Check sheet for the drawn part. Datum: minimum x, y, z corner. Units: mm. Round coordinates to 2 decimals unless told otherwise and drop trailing zeros. Order: outer loops, then holes, each group sorted by start corner. A loop starts at its lowest first (then second) coordinate and runs counter-clockwise, first axis right, second up. Notation, with made-up numbers: (-16, 65) -> (-8, 65) arc R25 ccw to (-8, 82) -> close; hole circle Ø11 at (62.5, 76.5). An arc over 180 degrees is marked (long way). Answer in a Markdown table with one row per item.
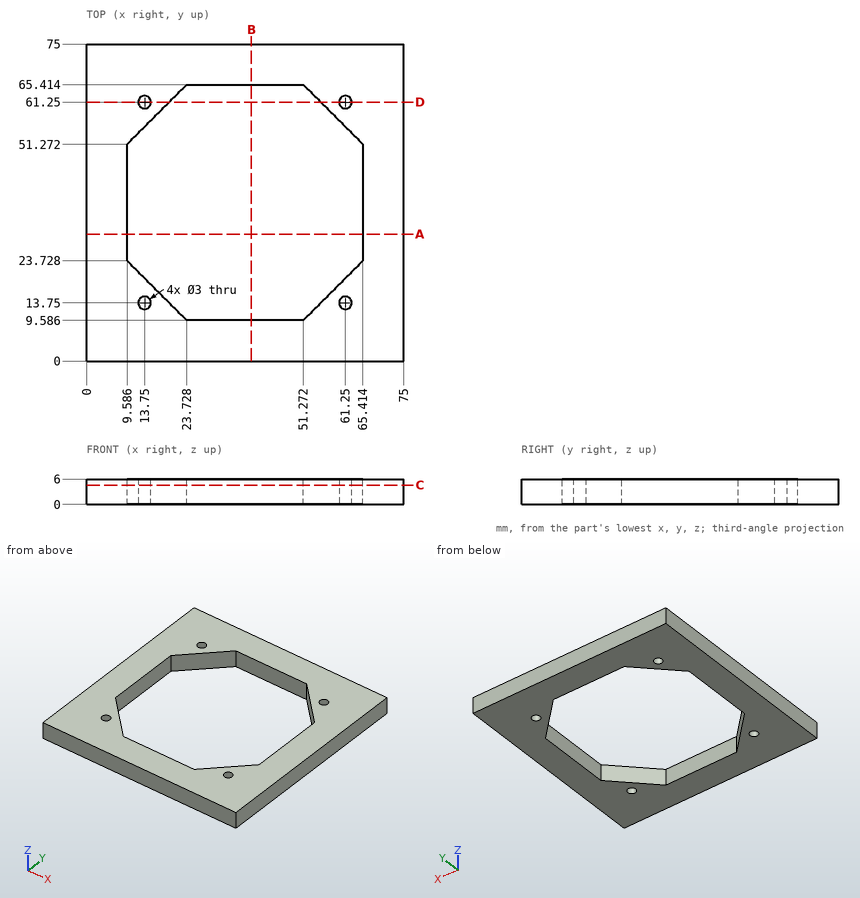
(1) Scan lines: probe 1 along X at (y, z) = (27, 2.4); probe 2 along Y at (x, z) = (61.5, 4.9). Record each from-to range of solid material in increasing order. Write a range as from..to.
Solutions:
| item | result |
|---|---|
| probe 1 | 0..9.59, 65.41..75 |
| probe 2 | 0..12.27, 15.23..19.81, 55.19..59.77, 62.73..75 |
(2) Section check A-A on y = 30. Record the boundary of the cut face in (x, z), plus the area to 3 significant figures.
Solutions:
| item | result |
|---|---|
| outline | (0, 0) -> (9.59, 0) -> (9.59, 6) -> (0, 6) -> close; (65.41, 0) -> (75, 0) -> (75, 6) -> (65.41, 6) -> close |
| area | 115 mm^2 |
(3) Section check D-D on y = 61.25. Record the boundary of the cut face in (x, z), plus the area to 3 significant figures.
Solutions:
| item | result |
|---|---|
| outline | (0, 0) -> (12.25, 0) -> (12.25, 6) -> (0, 6) -> close; (15.25, 0) -> (19.56, 0) -> (19.56, 6) -> (15.25, 6) -> close; (55.44, 0) -> (59.75, 0) -> (59.75, 6) -> (55.44, 6) -> close; (62.75, 0) -> (75, 0) -> (75, 6) -> (62.75, 6) -> close |
| area | 199 mm^2 |
(4) Section check C-C on z = 4.55. Record the boundary of the cut face in (x, y), plus the area to 3 significant figures.
Solutions:
| item | result |
|---|---|
| outline | (0, 0) -> (75, 0) -> (75, 75) -> (0, 75) -> close; hole (9.59, 23.73) -> (23.73, 9.59) -> (51.27, 9.59) -> (65.41, 23.73) -> (65.41, 51.27) -> (51.27, 65.41) -> (23.73, 65.41) -> (9.59, 51.27) -> close; hole circle Ø3 at (13.75, 13.75); hole circle Ø3 at (13.75, 61.25); hole circle Ø3 at (61.25, 13.75); hole circle Ø3 at (61.25, 61.25) |
| area | 2,880 mm^2 |
